Geometry: final body of the model. Coordinates: model frame, mm. Give positions to 0.01 mm unless a question says otherwise; leave off trailing zeros. Loops run counter-clockwise (first coordinate to the right, second up) from the corner with the lowest first, then second, coordinate; pieces in that order, holes last.
```python
from build123d import *

# Parameters (mm, degrees)
SKETCH2_R           = 20
SKETCH2_R_2         = 17.5
BOSS_EXTRUDE1_DEPTH = 650
SKETCH3_R           = 3
CUT_EXTRUDE1_DEPTH  = 30


with BuildPart() as part:
    # Sketch2 → Boss-Extrude1 (new body)
    with BuildSketch(Plane(origin=(0, 0, 0), x_dir=(0, 0, -1), z_dir=(1, 0, 0))):
        Circle(SKETCH2_R)
        Circle(SKETCH2_R_2, mode=Mode.SUBTRACT)
    extrude(amount=BOSS_EXTRUDE1_DEPTH)

    # Sketch3 → Cut-Extrude1 (cut, symmetric)
    with BuildSketch(Plane(origin=(0, 0, 0), x_dir=(1, 0, 0), z_dir=(0, 1, 0))):
        with Locations(Location((121.46797255, 2.5, 0), (0, 0, 270))):
            Circle(SKETCH3_R)
        with Locations(Location((521.46797255, 2.5, 0), (0, 0, 270))):
            Circle(SKETCH3_R)
    extrude(amount=CUT_EXTRUDE1_DEPTH, both=True, mode=Mode.SUBTRACT)


solid = part.part
```
Q1. Mould query, pull axis Z, two halves, no side actions, for faces 1 (the face through (320.45, -10.648, 13.887)), 2 (the face through (320.45, -19.524, 4.336)), 3 (the face through (650, -18, 0)). Classes: +Z half, -Z half, draft (parallel to the pull), parting line (faces both ways), or undercut.
Q2. Section query A-A, the plane y = 7. Return loops of the section in (x, z) (3 decimals), and give its area (3 significant figures).
Q3. Material intervals for probe 1 along X at (y, z) = (-18.1, -2.5); probe 2 along Z at (x, y) = (48, 1); probe 3 along Y at (x, z) = (226, 0), sorted ascending.
Q4. Pin query (flat end, axial travel): pin 1 Ø2 at (x, z) = (412.5, 3) entering from +Y; pin 2 Ø9.5 at (x, z) = (521.47, -2.5) entering from +Y; pin 3 Ø1.5 at (x, y) = (231.5, -5.5) entering from -Z; pin 4 Ø6 at (x, z) = (295.5, -3.5) entering from -Y. Return the tip coordinate at first contact, or that it passes through.
Q5. Section query B-B, the plane z = -12. Return loops of the section in (x, y), and give its area (3 significant figures).
Q6. Section query C-C, the plane x = 137. Return loops of the section in (y, z).
Resolved:
1. face 1: undercut
1. face 2: parting line
1. face 3: draft
2. outline: (0, -18.735) - (650, -18.735) - (650, -16.039) - (0, -16.039) - close; (0, 16.039) - (650, 16.039) - (650, 18.735) - (0, 18.735) - close
2. area: 3,500 mm2
3. probe 1: x = 0 to 118.47, 124.47 to 518.47, 524.47 to 650
3. probe 2: z = -19.97 to -17.47, 17.47 to 19.97
3. probe 3: y = -20 to -17.5, 17.5 to 20
4. pin 1: stops at y = 19.9
4. pin 2: stops at y = 20
4. pin 3: stops at z = -19.43
4. pin 4: stops at y = -19.99
5. outline: (0, -16) - (650, -16) - (650, -12.74) - (0, -12.74) - close; (0, 12.74) - (650, 12.74) - (650, 16) - (0, 16) - close
5. area: 4,240 mm2
6. outline: circle Ø40 at (0, 0); hole circle Ø35 at (0, 0)
